For this review, take the finished solid that the model builds, in its own axes (mm). Face numbers are marked on the shaded views. Coordinates: 2 decimals unless noted, no trailing zeros. Write each loop counter-clockwise with the first axis right and the second up, starting at its lowest first coordinate (ties: lowest second). Pieces come first, ordered by that corner, then holes.
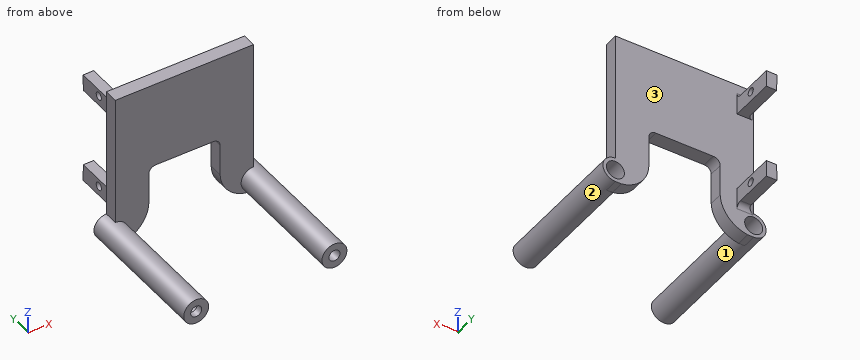
```python
from build123d import *

# Parameters (mm, degrees)
SKETCH1_R             = 3.6
SKETCH1_R_2           = 2.6
BOSS_EXTRUDE1_DEPTH   = 40
BOSS_EXTRUDE1_2_DEPTH = 40
BOSS_EXTRUDE2_START   = -4
BOSS_EXTRUDE2_DEPTH   = 4
SKETCH4_W             = 20.645
SKETCH4_H             = 20
CUT_EXTRUDE2_DEPTH    = 10
BOSS_EXTRUDE3_DEPTH   = 13
FILLET3_R             = 1.5
SKETCH6_R             = 1.135575656
SKETCH6_R_2           = 1.15
CUT_EXTRUDE3_DEPTH    = 13
FILLET4_R             = 2
SKETCH9_R             = 2.851630117
SKETCH9_R_2           = 1.6
BOSS_EXTRUDE4_DEPTH   = 2
SKETCH10_R            = 2.895791365
SKETCH10_R_2          = 1.6
BOSS_EXTRUDE5_DEPTH   = 4
CUT_EXTRUDE4_DEPTH    = 10


with BuildPart() as part:
    # Sketch1 → Boss-Extrude1 (new body)
    with BuildSketch(Plane(origin=(0, 0, 0), x_dir=(1, 0, 0), z_dir=(0, 1, 0))):
        with Locations(Location((-16.334138417, 4.403985818, 0), (0, 0, 270))):
            Circle(SKETCH1_R)
        with Locations(Location((-16.334138417, 4.403985818, 0), (0, 0, 270))):
            Circle(SKETCH1_R_2, mode=Mode.SUBTRACT)
    extrude(amount=BOSS_EXTRUDE1_DEPTH)



with BuildPart() as body_2:
    # Sketch1 → Boss-Extrude1 2 (new body)
    with BuildSketch(Plane(origin=(0, 0, 0), x_dir=(1, 0, 0), z_dir=(0, 1, 0))):
        with Locations(Location((23.665861583, 4.403985818, 0), (0, 0, 270))):
            Circle(SKETCH1_R)
        with Locations(Location((23.665861583, 4.403985818, 0), (0, 0, 270))):
            Circle(SKETCH1_R_2, mode=Mode.SUBTRACT)
    extrude(amount=BOSS_EXTRUDE1_2_DEPTH)


with BuildPart() as part_1:
    add(part.part)

    add(body_2.part)  # Boss-Extrude2 merges body 2
    # Sketch2 → Boss-Extrude2 (add)
    with BuildSketch(Plane(origin=(0, 40, 0), x_dir=(1, 0, 0), z_dir=(0, 1, 0)).offset(BOSS_EXTRUDE2_START)):
        with BuildLine():
            Line((-16.334138417, 8.003985818), (23.665861583, 8.003985818))
            ThreePointArc((23.665861583, 8.003985818), (20.065861583, 4.403985818), (23.665861583, 0.803985818))
            Line((23.665861583, 0.803985818), (23.665861583, -36.996014182))
            Line((23.665861583, -36.996014182), (-16.334138417, -36.996014182))
            Line((-16.334138417, -36.996014182), (-16.334138417, 0.803985818))
            ThreePointArc((-16.334138417, 0.803985818), (-12.734138417, 4.403985818), (-16.334138417, 8.003985818))
        make_face()
    extrude(amount=BOSS_EXTRUDE2_DEPTH)

    # Sketch4 → Cut-Extrude2 (cut)
    with BuildSketch(Plane(origin=(0, 40, 0), x_dir=(1, 0, 0), z_dir=(0, 1, 0))):
        with Locations((3.665861583, -1.996014182)):
            Rectangle(SKETCH4_W, SKETCH4_H)
    extrude(amount=-CUT_EXTRUDE2_DEPTH, mode=Mode.SUBTRACT)

    # Sketch5 → Boss-Extrude3 (add)
    with BuildSketch(Plane(origin=(0, 40, 0), x_dir=(1, 0, 0), z_dir=(0, 1, 0))):
        Polygon((-11.546638417, -5.036014182), (-14.546638417, -5.036014182), (-14.603209007, -0.236014182), (-11.546638417, -0.236014182), align=None)
        Polygon((-14.546638417, -28.036014182), (-11.546638417, -28.036014182), (-11.546638417, -32.836014182), (-14.603209007, -32.836014182), align=None)
    extrude(amount=BOSS_EXTRUDE3_DEPTH)

    # Fillet3
    fillet3_edges = [part_1.edges().sort_by_distance(p)[0] for p in [
        (-13.074923712, 40, 32.836014182),
        (-14.574923712, 40, 30.436014182),
        (-13.074923712, 40, 0.236014182),
        (-14.574923712, 40, 2.636014182),
    ]]
    fillet(fillet3_edges, radius=FILLET3_R)

    # Sketch6 → Cut-Extrude3 (cut)
    with BuildSketch(Plane(origin=(-11.546638417, 0.245033675, 0.24921506), x_dir=(0, 0, -1), z_dir=(1, 0, 0))):
        with Locations((-30.626521838, 45.832462835)):
            Circle(SKETCH6_R)
        with Locations((-2.699312308, 45.832462835)):
            Circle(SKETCH6_R_2)
    extrude(amount=-CUT_EXTRUDE3_DEPTH, mode=Mode.SUBTRACT)

    # Fillet4
    fillet4_edges = [part_1.edges().sort_by_distance(p)[0] for p in [
        (-6.656638417, 38, 11.996014182),
        (-6.656638417, 38, -8.003985818),
        (13.988361583, 38, -8.003985818),
        (13.988361583, 38, 11.996014182),
    ]]
    fillet(fillet4_edges, radius=FILLET4_R)

    # Sketch9 → Boss-Extrude4 (add)
    with BuildSketch(Plane.XZ):
        with Locations((-16.334138417, -4.403985818)):
            Circle(SKETCH9_R)
        with Locations(Location((-16.334138417, -4.403985818, 0), (0, 0, 270))):
            Circle(SKETCH9_R_2, mode=Mode.SUBTRACT)
    extrude(amount=-BOSS_EXTRUDE4_DEPTH)

    # Sketch10 → Boss-Extrude5 (add)
    with BuildSketch(Plane.XZ):
        with Locations((23.665861583, -4.403985818)):
            Circle(SKETCH10_R)
        with Locations(Location((23.665861583, -4.403985818, 0), (0, 0, 270))):
            Circle(SKETCH10_R_2, mode=Mode.SUBTRACT)
    extrude(amount=-BOSS_EXTRUDE5_DEPTH)

    # Sketch12 → Cut-Extrude4 (cut)
    with BuildSketch(Plane(origin=(0, 40, 0), x_dir=(1, 0, 0), z_dir=(0, 1, 0))):
        with BuildLine():
            Line((-14.597154628, 8.003985818), (-6.526218466, 8.003985818))
            Line((-6.526218466, 8.003985818), (-6.656638417, -0.894717181))
            ThreePointArc((-6.656638417, -0.894717181), (-9.013941955, 4.99391057), (-14.597154628, 8.003985818))
        make_face()
    cut_extrude4 = extrude(amount=-CUT_EXTRUDE4_DEPTH, mode=Mode.SUBTRACT)

    # Mirror1: Cut-Extrude4 across plane
    add(cut_extrude4.mirror(Plane.ZY.offset(-3.665861583)), mode=Mode.SUBTRACT)


solid = part_1.part
```
Q1. Add section B-B (y = 28). State the section outline as (x, z) points.
Ans:
outline: circle Ø7.2 at (-16.33, -4.4); circle Ø7.2 at (23.67, -4.4); hole circle Ø5.2 at (-16.33, -4.4); hole circle Ø5.2 at (23.67, -4.4)
Q2. Add section D-D (y = 49). State the section outline as (x, z) points, then the cut area to 3 significant figures.
Ans:
outline: (-14.6, 0.24) - (-11.55, 0.24) - (-11.55, 5.04) - (-14.55, 5.04) - close; (-14.6, 32.84) - (-14.55, 28.04) - (-11.55, 28.04) - (-11.55, 32.84) - close
area: 29.1 mm2
Q3. For probe 1 along X at (y, z) = (20.5, -5); probe 2 along Y at (x, z) = (-16, 24.5); probe 3 along Z at (x, y) = (-14, 14.5), list the stretches that pass through material, from the lowest coordinate up.
Ans:
probe 1: x = -19.88 to -18.86, -13.8 to -12.78, 20.12 to 21.14, 26.2 to 27.22
probe 2: y = 36 to 40
probe 3: z = -7.14 to -5.55, -3.26 to -1.66
Q4. Draft analysis for pull direction X (two halves, no side actions). For the marked faces 1, 2 and 3, state which applies: +X half, -X half, draft (parallel to the pull), parting line (faces both ways), or undercut.
Ans:
face 1: undercut
face 2: undercut
face 3: draft
Q5. Clearance check with flat-ended pins moving along their axes: pin 1 Ø3 at (y, z) = (37.5, 9.5) entering from -X; pin 2 Ø12 at (y, z) = (39.5, 2.5) entering from +X; pin 3 Ø1.2 at (x, y) = (4, 39) entering from -Z. State where each tip first meets the part, or that it passes through.
Ans:
pin 1: stops at x = -16.33
pin 2: stops at x = 27.15
pin 3: stops at z = 12
Q6. Add section A-A (y = 37). State the section outline as (x, z) points.
Ans:
outline: (-16.33, -8) - (-14.6, -8) arc R9.31 ccw to (-6.66, 0.89) - (-6.66, 10) arc R2 cw to (-4.66, 12) - (11.99, 12) arc R2 cw to (13.99, 10) - (13.99, 0.89) arc R9.31 ccw to (21.93, -8) - (23.67, -8) arc R3.6 ccw to (23.67, -0.8) - (23.67, 37) - (-16.33, 37) - (-16.33, -0.8) arc R3.6 ccw to start; hole circle Ø5.2 at (-16.33, -4.4); hole circle Ø5.2 at (23.67, -4.4)
Q7. Add section C-C (z = -5). State the section outline as (x, y) points.
Ans:
outline: (-19.88, 0) - (-17.82, 0) - (-17.82, 2) - (-18.86, 2) - (-18.86, 40) - (-19.88, 40) - close; (-14.85, 0) - (-12.78, 0) - (-12.78, 36) - (-9.02, 36) - (-9.02, 40) - (-13.8, 40) - (-13.8, 2) - (-14.85, 2) - close; (16.35, 36) - (20.12, 36) - (20.12, 0) - (22.18, 0) - (22.18, 4) - (21.14, 4) - (21.14, 40) - (16.35, 40) - close; (25.15, 0) - (27.22, 0) - (27.22, 40) - (26.2, 40) - (26.2, 4) - (25.15, 4) - close
